Here's how the part is built. I have some questions about the finished solid (model axes, mm). Face numbers are marked on the shaded views. A direction names the side the tool comes from. Coordinates: 2 decimals unless noted, no trailing zeros. Order: outer loops, then holes, each group sorted by start corner. A loop starts at its lowest first (then second) coordinate and runs counter-clockwise, first axis right, second up. Notation, with made-up numbers: (10, 55.5) - (48, 55.5) arc R21 ccw to (48, 62.5) - close; hole circle Ø11 at (83.5, 68). An arc over 180 degrees is marked (long way). Answer as CSV lines item,"result". Start each with the question number.
Q1. Suppose I cut it at A-A (x = 0). Please give me the cut outline in (y, z), then the cut area to 3 significant figures.
Q2. For pin 1 Ø4 at (x, z) = (6, 17.5) entering from +Y; pin 2 Ø1 at (x, y) = (-3, 6) entering from -Z; pin 3 Ø1.5 at (y, z) = (4, -0.5) entering from -X, each with a flat end and sliding along its axis, tell me the tip position at first contact or that it passes through.
Q3. Suppose I cut it at C-C (z = 23.5). Please give me the cut outline in (x, y).
Q4. For the marked faces 3 and 4, which set-ups out of +Z, -Z, +X, -X, +Y, -Y let a thin tool reach every point of the face, with its end or its side?
Q5. Thinking about a two-plate mould opening in X: for the marked faces 1 and 2, which applies, released by +X, released by -X, zero draft, split by the parting line, or undercut?
Q6. I need wall thicknesses on line 1 (Z direction, x = 0.25, y = -2.5); line 2 (X direction, y = -0.25, z = 14); line 3 (Y direction, x = 1.5, z = 35). Which ranges of each line are inside material? Lowest first, please.
Q7. Suppose I cut it at D-D (y = 6). Please give me the cut outline in (x, z).
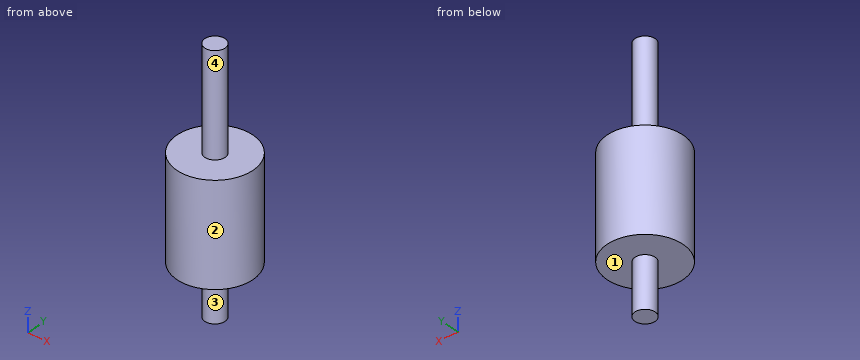
from build123d import *

# Parameters (mm, degrees)
SKETCH1_R                = 7.5
BOSS_EXTRUDE1_DEPTH      = 20
SKETCH2_R                = 1
BOSS_EXTRUDE3_DEPTH      = 40
BOSS_EXTRUDE3_DEPTH_BACK = 10
SKETCH3_R                = 2
BOSS_EXTRUDE4_DEPTH      = 40
BOSS_EXTRUDE4_DEPTH_BACK = 10


with BuildPart() as part:
    # Sketch1 → Boss-Extrude1 (new body)
    with BuildSketch(Plane.XY):
        Circle(SKETCH1_R)
    extrude(amount=BOSS_EXTRUDE1_DEPTH)

    # Sketch2 → Boss-Extrude3 (add, two sides)
    with BuildSketch(Plane.XY) as boss_extrude3_sk:
        Circle(SKETCH2_R)
    extrude(amount=BOSS_EXTRUDE3_DEPTH)
    extrude(boss_extrude3_sk.sketch, amount=-BOSS_EXTRUDE3_DEPTH_BACK)

    # Sketch3 → Boss-Extrude4 (add, two sides)
    with BuildSketch(Plane.XY) as boss_extrude4_sk:
        Circle(SKETCH3_R)
    extrude(amount=BOSS_EXTRUDE4_DEPTH)
    extrude(boss_extrude4_sk.sketch, amount=-BOSS_EXTRUDE4_DEPTH_BACK)


solid = part.part
Here are the results:
1,outline,"(-7.5, 0) - (-2, 0) - (-2, -10) - (2, -10) - (2, 0) - (7.5, 0) - (7.5, 20) - (2, 20) - (2, 40) - (-2, 40) - (-2, 20) - (-7.5, 20) - close"
1,area,"420 mm²"
2,pin 1,"stops at y = 6.34"
2,pin 2,"stops at z = 0"
2,pin 3,"stops at x = -6.66"
3,outline,"circle Ø4 at (0, 0)"
4,face 3,"-Z"
4,face 4,"+Z"
5,face 1,"zero draft"
5,face 2,"split by the parting line"
6,line 1,"z = 0 to 20"
6,line 2,"x = -7.5 to 7.5"
6,line 3,"y = -1.32 to 1.32"
7,outline,"(-4.5, 0) - (4.5, 0) - (4.5, 20) - (-4.5, 20) - close"
